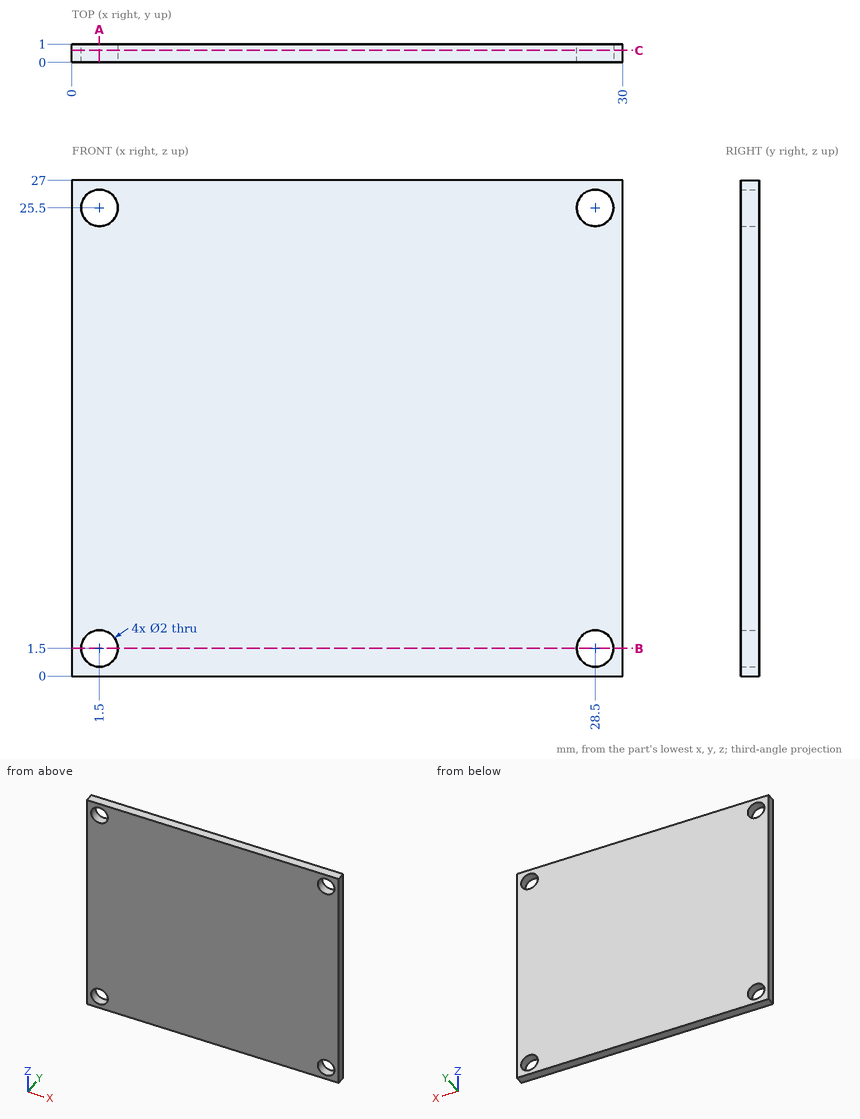
The drawing under review shows one solid part. Ordinate dimensions are in mm from its lowest x, y, z. Round coordinates to 2 decimals unless told otherwise and drop trailing zeros. Loops run counter-clockwise (first coordinate to the right, second up) from the corner with the lowest first, then second, coordinate; pieces in that order, holes last. Notation, with made-up numbers: (-26.5, -1.75) - (5.5, -1.75) arc R5 ccw to (5.5, 3.25) - close; hole circle Ø3 at (-3.75, 62.5). An arc over 180 degrees is marked (long way). Use a Markdown table: item, result. Add a question column.
Q1. For probe 1 along Z at (x, y) = (1.5, 0.35); probe 2 along X at (y, z) = (0.3, 1.5); probe 3 along X at (y, z) = (0.6, 2), list the stretches that pass through material, from the lowest coordinate up.
Q2. Add section A-A (x = 1.5). State the section outline as (y, z) points.
Q3. Add section B-B (z = 1.5). State the section outline as (x, y) points.
Q4. Add section C-C (y = 0.65). State the section outline as (x, z) points.
Worked answers:
| question | item | result |
|---|---|---|
| 1 | probe 1 | 0 to 0.5, 2.5 to 24.5, 26.5 to 27 |
| 1 | probe 2 | 0 to 0.5, 2.5 to 27.5, 29.5 to 30 |
| 1 | probe 3 | 0 to 0.63, 2.37 to 27.63, 29.37 to 30 |
| 2 | outline | (0, 0) - (1, 0) - (1, 0.5) - (0, 0.5) - close; (0, 2.5) - (1, 2.5) - (1, 24.5) - (0, 24.5) - close; (0, 26.5) - (1, 26.5) - (1, 27) - (0, 27) - close |
| 3 | outline | (0, 0) - (0.5, 0) - (0.5, 1) - (0, 1) - close; (2.5, 0) - (27.5, 0) - (27.5, 1) - (2.5, 1) - close; (29.5, 0) - (30, 0) - (30, 1) - (29.5, 1) - close |
| 4 | outline | (0, 0) - (30, 0) - (30, 27) - (0, 27) - close; hole circle Ø2 at (1.5, 1.5); hole circle Ø2 at (1.5, 25.5); hole circle Ø2 at (28.5, 1.5); hole circle Ø2 at (28.5, 25.5) |
